CAD build for the part. Positions are in the model's coordinates, mm. A direction names the side the tool comes from. Give positions to 0.01 mm unless a question says otherwise; leave off trailing zeros. Order: outer loops, then holes, each group sorted by start corner. A loop starts at its lowest first (then second) coordinate and runs counter-clockwise, first axis right, second up.
Item 1: Band-saw the part on C-C on x = 127. Give the cut face in (y, z) (3 decimals), plus the area to 3 significant figures.
Item 2: Band-saw the part on A-A on x = 25.4. Give the cut face in (y, z) (3 decimals).
Item 3: Which spindle directions (+Z, -Z, +X, -X, +Y, -Y) get a long thin tool onto all of the face, cutting with end or side? Do faces 4 (the flat face through (70, 29, 9.525)), 5 (the cylindrical face through (98.501, 50.711, 6.806)). Say none if no direction does.
Item 4: Band-saw the part on B-B on y = 26. Give the cut face in (x, z) (1 decimal), plus the area to 3 significant figures.
Item 5: Band-saw the part on D-D on z = 1.5. Give the cut face in (x, y) (3 decimals), plus the area to 3 significant figures.
Item 6: Two-plate mould, pull along X, no slides. Class faces 1 (the cylindrical face through (23.93, 44.81, 4.7)), 2 (the cylindrical face through (142.87, 27.95, 4.7)), 3 (the flat face through (70, 29, 0)): released by +X, released by -X, zero draft, split by the parting line, or undercut.
Item 7: Wall check: L1, parallel to Y at x = 25.4, z = 4; L2, parallel to X at y = 47.75, z = 5.08; L3, parallel to X at y = 46.5, z = 1.5. Give the ranges that are in metal, low to high.
Item 8: Flat gauge pins, fed straight in: P1, Ø1.5, axis at y = 26, z = 3.5, coming from the +X side; P2, Ø2, axis at x = 117.5, z = 3.5, coming from the -Y side. Where does each tip first touch, or does it go through?
```python
from build123d import *

# Parameters (mm, degrees)
BOSS_EXTRUDE1_DEPTH         = 9.525
F_5_8_18_TAPPED_HOLE1_D     = 14.68374
F_1_4_0_25_DIAMETER_HOLE1_D = 6.35
F_8_32_TAPPED_HOLE1_D       = 3.4544
F_8_32_TAPPED_HOLE1_DEPTH   = 12.7
F_8_32_TAPPED_HOLE1_TIP     = 1.037806461


with BuildPart() as part:
    # Sketch1 → Boss-Extrude1 (new body)
    with BuildSketch(Plane.XY):
        with BuildLine():
            Line((0, 0), (114.3, 0))
            ThreePointArc((114.3, 0), (142.875, 28.575), (114.3, 57.15))
            Line((114.3, 57.15), (0, 57.15))
            Line((0, 57.15), (0, 0))
        make_face()
    extrude(amount=BOSS_EXTRUDE1_DEPTH)

    # 5/8-18 Tapped Hole1 (through all)
    with Locations(Plane.XY.offset(9.525)):
        with Locations((127, 28.575)):
            Hole(F_5_8_18_TAPPED_HOLE1_D / 2)

    # 1/4 (0.25) Diameter Hole1 (through all)
    with Locations(Plane(origin=(25.4, 47.625, 9.525), x_dir=(1, 0, 0), z_dir=(0, 0, 1))):
        with Locations((0, 0), (0, -38.1)):
            Hole(F_1_4_0_25_DIAMETER_HOLE1_D / 2)

    # #8-32 Tapped Hole1
    with Locations(Plane(origin=(98.425, 57.15, 5.08), x_dir=(0, 0, 1), z_dir=(0, 1, 0))):
        with Locations((0, 0)):
            Hole(F_8_32_TAPPED_HOLE1_D / 2, depth=F_8_32_TAPPED_HOLE1_DEPTH)
            with Locations((0, 0, -(F_8_32_TAPPED_HOLE1_DEPTH + F_8_32_TAPPED_HOLE1_TIP / 2))):  # 118° drill point
                Cone(0, F_8_32_TAPPED_HOLE1_D / 2, F_8_32_TAPPED_HOLE1_TIP, mode=Mode.SUBTRACT)


solid = part.part
```
The answers:
1. outline: (2.977, 0) - (21.233, 0) - (21.233, 9.525) - (2.977, 9.525) - close; (35.917, 0) - (54.173, 0) - (54.173, 9.525) - (35.917, 9.525) - close
1. area: 348 mm2
2. outline: (0, 0) - (6.35, 0) - (6.35, 9.525) - (0, 9.525) - close; (12.7, 0) - (44.45, 0) - (44.45, 9.525) - (12.7, 9.525) - close; (50.8, 0) - (57.15, 0) - (57.15, 9.525) - (50.8, 9.525) - close
3. face 4: +Z, +X, -X, +Y, -Y
3. face 5: +Y
4. outline: (0, 0) - (120.1, 0) - (120.1, 9.5) - (0, 9.5) - close; (133.9, 0) - (142.8, 0) - (142.8, 9.5) - (133.9, 9.5) - close
4. area: 1,230 mm2
5. outline: (0, 0) - (114.3, 0) arc R28.575 ccw to (114.3, 57.15) - (0, 57.15) - close; hole circle Ø6.35 at (25.4, 9.525); hole circle Ø6.35 at (25.4, 47.625); hole circle Ø14.684 at (127, 28.575)
5. area: 7,580 mm2
6. face 1: undercut
6. face 2: released by +X
6. face 3: zero draft
7. L1: y = 0 to 6.35, 12.7 to 44.45, 50.8 to 57.15
7. L2: x = 0 to 22.23, 28.57 to 96.7, 100.15 to 135.49
7. L3: x = 0 to 22.43, 28.37 to 136.55
8. P1: stops at x = 142.82
8. P2: stops at y = 0.08
